Source: CAD feature listing. Evaluate the final solid. Frame: model axes, mm. Coordinates: 2 decimals unless noted, no trailing zeros. Write each loop counter-clockwise with the first axis right and the second up, starting at its lowest first coordinate (ties: lowest second). Pieces come first, ordered by that corner, then holes. Notation, with made-up numbers: (42.25, 2.25) - (65.25, 2.25) arc R33 cw to (65.25, 39.25) - close; hole circle Ø3 at (42.25, -5). An arc over 180 degrees is marked (long way). One line per question, with ' | ' between items.
Autodesk Inventor part; units mm, degrees
ref_plane "YZ Plane" through (0, 0, 0) normal (1, 0, 0) x (0, 1, 0)
ref_plane "XZ Plane" through (0, 0, 0) normal (0, 1, 0) x (-1, 0, 0)
ref_plane "XY Plane" through (0, 0, 0) normal (0, 0, 1) x (1, 0, 0)
sketch "Sketch1" plane through (0, 0, 0) normal (0, 1, 0) x (-1, 0, 0)
  line L0 (42.7926, 25.861) -> (42.8013, 25.866)
  line L1 (43.7926, 24.129) -> (43.8013, 24.134)
  line L2 (1, 50) -> (1, 49.99)
  line L3 (-1, 50) -> (-1, 49.99)
  line L4 (42.7926, -25.861) -> (42.8013, -25.866)
  line L5 (43.7926, -24.129) -> (43.8013, -24.134)
  line L6 (1, -49.99) -> (1, -50)
  line L7 (-1, -49.99) -> (-1, -50)
  line L8 (-42.8013, -25.866) -> (-42.7926, -25.861)
  line L9 (-43.8013, -24.134) -> (-43.7926, -24.129)
  line L10 (-43.8013, 24.134) -> (-43.7926, 24.129)
  line L11 (-42.8013, 25.866) -> (-42.7926, 25.861)
  line L12 (4.7426, 1.5835) -> (43.7926, 24.129)
  line L13 (4.7426, -1.5835) -> (43.7926, -24.129)
  line L14 (1, 49.99) -> (1, 4.899)
  line L15 (3.7426, 3.3155) -> (42.7926, 25.861)
  line L16 (-42.7926, 25.861) -> (-3.7426, 3.3155)
  line L17 (-1, 49.99) -> (-1, 4.899)
  line L18 (-43.7926, -24.129) -> (-4.7426, -1.5835)
  line L19 (-43.7926, 24.129) -> (-4.7426, 1.5835)
  line L20 (-42.7926, -25.861) -> (-3.7426, -3.3155)
  line L21 (-1, -4.899) -> (-1, -49.99)
  line L22 (3.7426, -3.3155) -> (42.7926, -25.861)
  line L23 (1, -4.899) -> (1, -49.99)
  circle A0 centre (0, 0) radius 52
  arc A1 (-1, 49.99) -> (-42.7926, 25.861) centre (0, 0) ccw
  arc A2 (-43.7926, 24.129) -> (-43.7926, -24.129) centre (0, 0) ccw
  arc A3 (-42.7926, -25.861) -> (-1, -49.99) centre (0, 0) ccw
  arc A4 (1, -49.99) -> (42.7926, -25.861) centre (0, 0) ccw
  arc A5 (43.7926, -24.129) -> (43.7926, 24.129) centre (0, 0) ccw
  arc A6 (42.7926, 25.861) -> (1, 49.99) centre (0, 0) ccw
  arc A7 (1, -4.899) -> (3.7426, -3.3155) centre (0, 0) ccw
  arc A8 (-3.7426, -3.3155) -> (-1, -4.899) centre (0, 0) ccw
  arc A9 (-4.7426, 1.5835) -> (-4.7426, -1.5835) centre (0, 0) ccw
  arc A10 (-1, 4.899) -> (-3.7426, 3.3155) centre (0, 0) ccw
  arc A11 (4.7426, -1.5835) -> (4.7426, 1.5835) centre (0, 0) ccw
  arc A12 (3.7426, 3.3155) -> (1, 4.899) centre (0, 0) ccw
extrude "Extrusion1" add sketch "Sketch1" along normal blind 50
properties part number "wheel"
Item 1: Mould query, pull axis Z, two halves, no side actions, for faces 1 (the face through (-24, 24.6, 12.7)), 2 (the face through (0, 50, 0)). Classes: pulls with the +Z half, pulls with the -Z half, needs draft (parallel to the pull), parting line crosses it, or undercut.
Check sheet entries:
face 1: undercut | face 2: needs draft
Item 2: Pin query (flat end, axial travel): pin 1 Ø13.5 at (y, z) = (15.5, 32.5) entering from +X; pin 2 Ø13.5 at (y, z) = (14.5, -31) entering from -X; pin 3 Ø22.5 at (y, z) = (18, 29.5) entering from -X. Return the tip coordinate at first contact, or that it passes through.
Check sheet entries:
pin 1: x = 45.18 | pin 2: x = -46 | pin 3: x = -48.69
Item 3: Cut plane D-D on z = -31. Return loops of the section in (x, y), and give its area (3 significant figures).
Check sheet entries:
outline: (-41.75, 0) - (-39.23, 0) - (-39.23, 50) - (-41.75, 50) - close; (-1, 0) - (1, 0) - (1, 50) - (-1, 50) - close; (39.23, 0) - (41.75, 0) - (41.75, 50) - (39.23, 50) - close | area: 352 mm²
Item 4: Cut plane C-C on x = -7. Return loops of the section in (y, z).
Check sheet entries:
outline: (0, -51.53) - (50, -51.53) - (50, -49.51) - (0, -49.51) - close; (0, -5.2) - (50, -5.2) - (50, -2.89) - (0, -2.89) - close; (0, 2.89) - (50, 2.89) - (50, 5.2) - (0, 5.2) - close; (0, 49.51) - (50, 49.51) - (50, 51.53) - (0, 51.53) - close
Item 5: Cut plane A-A on z = 0. Return loops of the section in (x, y).
Check sheet entries:
outline: (-52, 0) - (-50, 0) - (-50, 50) - (-52, 50) - close; (-5, 0) - (5, 0) - (5, 50) - (-5, 50) - close; (50, 0) - (52, 0) - (52, 50) - (50, 50) - close
Item 6: Ray query, line 1 along X through (y, z) = (29, -1); line 2 along Z through (x, y) = (22, 8.5); line 3 along Z through (x, y) = (-13.5, 21.5). Return the intervals inside material, ascending. Write a range as [from, to].
Check sheet entries:
line 1: [-51.99, -49.99], [-4.9, 4.9], [49.99, 51.99] | line 2: [-47.12, -44.9], [-13.86, -11.55], [11.55, 13.86], [44.9, 47.12] | line 3: [-50.22, -48.14], [-8.95, -6.64], [6.64, 8.95], [48.14, 50.22]
Item 7: Cut plane B-B on y = 13. Return loops of the section in (x, z).
Check sheet entries:
outline: circle Ø104 at (0, 0); hole (-43.79, -24.13) - (-4.74, -1.58) arc R5 cw to (-4.74, 1.58) - (-43.79, 24.13) arc R50 ccw to start; hole (-42.79, -25.86) arc R50 ccw to (-1, -49.99) - (-1, -4.9) arc R5 cw to (-3.74, -3.32) - close; hole (-42.79, 25.86) - (-3.74, 3.32) arc R5 cw to (-1, 4.9) - (-1, 49.99) arc R50 ccw to start; hole (1, -49.99) arc R50 ccw to (42.79, -25.86) - (3.74, -3.32) arc R5 cw to (1, -4.9) - close; hole (1, 4.9) arc R5 cw to (3.74, 3.32) - (42.79, 25.86) arc R50 ccw to (1, 49.99) - close; hole (4.74, -1.58) - (43.79, -24.13) arc R50 ccw to (43.79, 24.13) - (4.74, 1.58) arc R5 cw to start
